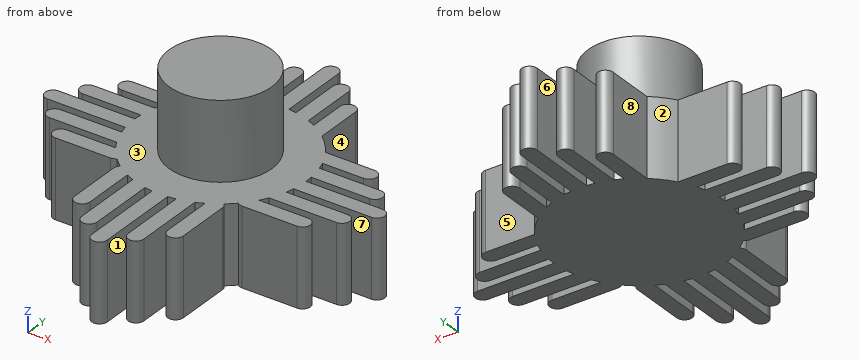
```python
from build123d import *

# Parameters (mm, degrees)
BOSS_EXTRUDE3_DEPTH    = 10
BOSS_EXTRUDE3_2_DEPTH  = 10
BOSS_EXTRUDE3_3_DEPTH  = 10
BOSS_EXTRUDE3_4_DEPTH  = 10
BOSS_EXTRUDE3_5_DEPTH  = 10
BOSS_EXTRUDE3_6_DEPTH  = 10
BOSS_EXTRUDE3_7_DEPTH  = 10
BOSS_EXTRUDE3_8_DEPTH  = 10
BOSS_EXTRUDE3_9_DEPTH  = 10
BOSS_EXTRUDE3_10_DEPTH = 10
BOSS_EXTRUDE3_11_DEPTH = 10
BOSS_EXTRUDE3_12_DEPTH = 10
BOSS_EXTRUDE3_13_DEPTH = 10
BOSS_EXTRUDE3_14_DEPTH = 10
BOSS_EXTRUDE3_15_DEPTH = 10
BOSS_EXTRUDE3_16_DEPTH = 10
BOSS_EXTRUDE3_17_DEPTH = 10
BOSS_EXTRUDE3_18_DEPTH = 10
BOSS_EXTRUDE3_19_DEPTH = 10
BOSS_EXTRUDE3_20_DEPTH = 10
SKETCH12_R             = 11
BOSS_EXTRUDE4_DEPTH    = 10
SKETCH13_R             = 6.585
BOSS_EXTRUDE5_DEPTH    = 10


with BuildPart() as part:
    # Sketch11 → Boss-Extrude3 (new body)
    with BuildSketch(Plane.XY):
        with BuildLine():
            Line((24.4, 31.507143862), (24.4, 46.249205315))
            ThreePointArc((24.4, 46.249205315), (25.4, 47.249205315), (26.4, 46.249205315))
            Line((26.4, 46.249205315), (26.4, 31.507143862))
            ThreePointArc((26.4, 31.507143862), (25.4, 30.507143862), (24.4, 31.507143862))
        make_face()
    extrude(amount=BOSS_EXTRUDE3_DEPTH)



with BuildPart() as body_2:
    # Sketch11 → Boss-Extrude3 2 (new body)
    with BuildSketch(Plane.XY):
        with BuildLine():
            Line((27.4, 30.400840206), (27.4, 43.867696771))
            ThreePointArc((27.4, 43.867696771), (28.4, 44.867696771), (29.4, 43.867696771))
            Line((29.4, 43.867696771), (29.4, 30.400840206))
            ThreePointArc((29.4, 30.400840206), (28.4, 29.400840206), (27.4, 30.400840206))
        make_face()
    extrude(amount=BOSS_EXTRUDE3_2_DEPTH)


with BuildPart() as body_3:
    # Sketch11 → Boss-Extrude3 3 (new body)
    with BuildSketch(Plane.XY):
        with BuildLine():
            Line((30.4, 33.885281374), (30.4, 40.954829552))
            ThreePointArc((30.4, 40.954829552), (31.4, 41.954829552), (32.4, 40.954829552))
            Line((32.4, 40.954829552), (32.4, 33.885281374))
            ThreePointArc((32.4, 33.885281374), (31.4, 32.885281374), (30.4, 33.885281374))
        make_face()
    extrude(amount=BOSS_EXTRUDE3_3_DEPTH)


with BuildPart() as body_4:
    # Sketch11 → Boss-Extrude3 4 (new body)
    with BuildSketch(Plane.XY):
        with BuildLine():
            Line((23.4, 30.400840206), (23.4, 43.867696771))
            ThreePointArc((23.4, 43.867696771), (22.4, 44.867696771), (21.4, 43.867696771))
            Line((21.4, 43.867696771), (21.4, 30.400840206))
            ThreePointArc((21.4, 30.400840206), (22.4, 29.400840206), (23.4, 30.400840206))
        make_face()
    extrude(amount=BOSS_EXTRUDE3_4_DEPTH)


with BuildPart() as body_5:
    # Sketch11 → Boss-Extrude3 5 (new body)
    with BuildSketch(Plane.XY):
        with BuildLine():
            Line((20.4, 33.885281374), (20.4, 40.954829552))
            ThreePointArc((20.4, 40.954829552), (19.4, 41.954829552), (18.4, 40.954829552))
            Line((18.4, 40.954829552), (18.4, 33.885281374))
            ThreePointArc((18.4, 33.885281374), (19.4, 32.885281374), (20.4, 33.885281374))
        make_face()
    extrude(amount=BOSS_EXTRUDE3_5_DEPTH)


with BuildPart() as body_6:
    # Sketch11 → Boss-Extrude3 6 (new body)
    with BuildSketch(Plane.XY):
        with BuildLine():
            Line((31.507143862, 26.4), (46.249205315, 26.4))
            ThreePointArc((46.249205315, 26.4), (47.249205315, 25.4), (46.249205315, 24.4))
            Line((46.249205315, 24.4), (31.507143862, 24.4))
            ThreePointArc((31.507143862, 24.4), (30.507143862, 25.4), (31.507143862, 26.4))
        make_face()
    extrude(amount=BOSS_EXTRUDE3_6_DEPTH)


with BuildPart() as body_7:
    # Sketch11 → Boss-Extrude3 7 (new body)
    with BuildSketch(Plane.XY):
        with BuildLine():
            Line((30.400840206, 23.4), (43.867696771, 23.4))
            ThreePointArc((43.867696771, 23.4), (44.867696771, 22.4), (43.867696771, 21.4))
            Line((43.867696771, 21.4), (30.400840206, 21.4))
            ThreePointArc((30.400840206, 21.4), (29.400840206, 22.4), (30.400840206, 23.4))
        make_face()
    extrude(amount=BOSS_EXTRUDE3_7_DEPTH)


with BuildPart() as body_8:
    # Sketch11 → Boss-Extrude3 8 (new body)
    with BuildSketch(Plane.XY):
        with BuildLine():
            Line((33.885281374, 20.4), (40.954829552, 20.4))
            ThreePointArc((40.954829552, 20.4), (41.954829552, 19.4), (40.954829552, 18.4))
            Line((40.954829552, 18.4), (33.885281374, 18.4))
            ThreePointArc((33.885281374, 18.4), (32.885281374, 19.4), (33.885281374, 20.4))
        make_face()
    extrude(amount=BOSS_EXTRUDE3_8_DEPTH)


with BuildPart() as body_9:
    # Sketch11 → Boss-Extrude3 9 (new body)
    with BuildSketch(Plane.XY):
        with BuildLine():
            Line((30.400840206, 27.4), (43.867696771, 27.4))
            ThreePointArc((43.867696771, 27.4), (44.867696771, 28.4), (43.867696771, 29.4))
            Line((43.867696771, 29.4), (30.400840206, 29.4))
            ThreePointArc((30.400840206, 29.4), (29.400840206, 28.4), (30.400840206, 27.4))
        make_face()
    extrude(amount=BOSS_EXTRUDE3_9_DEPTH)


with BuildPart() as body_10:
    # Sketch11 → Boss-Extrude3 10 (new body)
    with BuildSketch(Plane.XY):
        with BuildLine():
            Line((33.885281374, 30.4), (40.954829552, 30.4))
            ThreePointArc((40.954829552, 30.4), (41.954829552, 31.4), (40.954829552, 32.4))
            Line((40.954829552, 32.4), (33.885281374, 32.4))
            ThreePointArc((33.885281374, 32.4), (32.885281374, 31.4), (33.885281374, 30.4))
        make_face()
    extrude(amount=BOSS_EXTRUDE3_10_DEPTH)


with BuildPart() as body_11:
    # Sketch11 → Boss-Extrude3 11 (new body)
    with BuildSketch(Plane.XY):
        with BuildLine():
            Line((26.4, 19.292856138), (26.4, 4.550794685))
            ThreePointArc((26.4, 4.550794685), (25.4, 3.550794685), (24.4, 4.550794685))
            Line((24.4, 4.550794685), (24.4, 19.292856138))
            ThreePointArc((24.4, 19.292856138), (25.4, 20.292856138), (26.4, 19.292856138))
        make_face()
    extrude(amount=BOSS_EXTRUDE3_11_DEPTH)


with BuildPart() as body_12:
    # Sketch11 → Boss-Extrude3 12 (new body)
    with BuildSketch(Plane.XY):
        with BuildLine():
            Line((23.4, 20.399159794), (23.4, 6.932303229))
            ThreePointArc((23.4, 6.932303229), (22.4, 5.932303229), (21.4, 6.932303229))
            Line((21.4, 6.932303229), (21.4, 20.399159794))
            ThreePointArc((21.4, 20.399159794), (22.4, 21.399159794), (23.4, 20.399159794))
        make_face()
    extrude(amount=BOSS_EXTRUDE3_12_DEPTH)


with BuildPart() as body_13:
    # Sketch11 → Boss-Extrude3 13 (new body)
    with BuildSketch(Plane.XY):
        with BuildLine():
            Line((20.4, 16.914718626), (20.4, 9.845170448))
            ThreePointArc((20.4, 9.845170448), (19.4, 8.845170448), (18.4, 9.845170448))
            Line((18.4, 9.845170448), (18.4, 16.914718626))
            ThreePointArc((18.4, 16.914718626), (19.4, 17.914718626), (20.4, 16.914718626))
        make_face()
    extrude(amount=BOSS_EXTRUDE3_13_DEPTH)


with BuildPart() as body_14:
    # Sketch11 → Boss-Extrude3 14 (new body)
    with BuildSketch(Plane.XY):
        with BuildLine():
            Line((27.4, 20.399159794), (27.4, 6.932303229))
            ThreePointArc((27.4, 6.932303229), (28.4, 5.932303229), (29.4, 6.932303229))
            Line((29.4, 6.932303229), (29.4, 20.399159794))
            ThreePointArc((29.4, 20.399159794), (28.4, 21.399159794), (27.4, 20.399159794))
        make_face()
    extrude(amount=BOSS_EXTRUDE3_14_DEPTH)


with BuildPart() as body_15:
    # Sketch11 → Boss-Extrude3 15 (new body)
    with BuildSketch(Plane.XY):
        with BuildLine():
            Line((30.4, 16.914718626), (30.4, 9.845170448))
            ThreePointArc((30.4, 9.845170448), (31.4, 8.845170448), (32.4, 9.845170448))
            Line((32.4, 9.845170448), (32.4, 16.914718626))
            ThreePointArc((32.4, 16.914718626), (31.4, 17.914718626), (30.4, 16.914718626))
        make_face()
    extrude(amount=BOSS_EXTRUDE3_15_DEPTH)


with BuildPart() as body_16:
    # Sketch11 → Boss-Extrude3 16 (new body)
    with BuildSketch(Plane.XY):
        with BuildLine():
            Line((19.292856138, 24.4), (4.550794685, 24.4))
            ThreePointArc((4.550794685, 24.4), (3.550794685, 25.4), (4.550794685, 26.4))
            Line((4.550794685, 26.4), (19.292856138, 26.4))
            ThreePointArc((19.292856138, 26.4), (20.292856138, 25.4), (19.292856138, 24.4))
        make_face()
    extrude(amount=BOSS_EXTRUDE3_16_DEPTH)


with BuildPart() as body_17:
    # Sketch11 → Boss-Extrude3 17 (new body)
    with BuildSketch(Plane.XY):
        with BuildLine():
            Line((20.399159794, 27.4), (6.932303229, 27.4))
            ThreePointArc((6.932303229, 27.4), (5.932303229, 28.4), (6.932303229, 29.4))
            Line((6.932303229, 29.4), (20.399159794, 29.4))
            ThreePointArc((20.399159794, 29.4), (21.399159794, 28.4), (20.399159794, 27.4))
        make_face()
    extrude(amount=BOSS_EXTRUDE3_17_DEPTH)


with BuildPart() as body_18:
    # Sketch11 → Boss-Extrude3 18 (new body)
    with BuildSketch(Plane.XY):
        with BuildLine():
            Line((16.914718626, 30.4), (9.845170448, 30.4))
            ThreePointArc((9.845170448, 30.4), (8.845170448, 31.4), (9.845170448, 32.4))
            Line((9.845170448, 32.4), (16.914718626, 32.4))
            ThreePointArc((16.914718626, 32.4), (17.914718626, 31.4), (16.914718626, 30.4))
        make_face()
    extrude(amount=BOSS_EXTRUDE3_18_DEPTH)


with BuildPart() as body_19:
    # Sketch11 → Boss-Extrude3 19 (new body)
    with BuildSketch(Plane.XY):
        with BuildLine():
            Line((20.399159794, 23.4), (6.932303229, 23.4))
            ThreePointArc((6.932303229, 23.4), (5.932303229, 22.4), (6.932303229, 21.4))
            Line((6.932303229, 21.4), (20.399159794, 21.4))
            ThreePointArc((20.399159794, 21.4), (21.399159794, 22.4), (20.399159794, 23.4))
        make_face()
    extrude(amount=BOSS_EXTRUDE3_19_DEPTH)


with BuildPart() as body_20:
    # Sketch11 → Boss-Extrude3 20 (new body)
    with BuildSketch(Plane.XY):
        with BuildLine():
            Line((16.914718626, 20.4), (9.845170448, 20.4))
            ThreePointArc((9.845170448, 20.4), (8.845170448, 19.4), (9.845170448, 18.4))
            Line((9.845170448, 18.4), (16.914718626, 18.4))
            ThreePointArc((16.914718626, 18.4), (17.914718626, 19.4), (16.914718626, 20.4))
        make_face()
    extrude(amount=BOSS_EXTRUDE3_20_DEPTH)


with BuildPart() as part_1:
    add(part.part)

    add(body_2.part)  # Boss-Extrude4 merges body 2

    add(body_3.part)  # Boss-Extrude4 merges body 3

    add(body_4.part)  # Boss-Extrude4 merges body 4

    add(body_5.part)  # Boss-Extrude4 merges body 5

    add(body_6.part)  # Boss-Extrude4 merges body 6

    add(body_7.part)  # Boss-Extrude4 merges body 7

    add(body_8.part)  # Boss-Extrude4 merges body 8

    add(body_9.part)  # Boss-Extrude4 merges body 9

    add(body_10.part)  # Boss-Extrude4 merges body 10

    add(body_11.part)  # Boss-Extrude4 merges body 11

    add(body_12.part)  # Boss-Extrude4 merges body 12

    add(body_13.part)  # Boss-Extrude4 merges body 13

    add(body_14.part)  # Boss-Extrude4 merges body 14

    add(body_15.part)  # Boss-Extrude4 merges body 15

    add(body_16.part)  # Boss-Extrude4 merges body 16

    add(body_17.part)  # Boss-Extrude4 merges body 17

    add(body_18.part)  # Boss-Extrude4 merges body 18

    add(body_19.part)  # Boss-Extrude4 merges body 19

    add(body_20.part)  # Boss-Extrude4 merges body 20
    # Sketch12 → Boss-Extrude4 (add)
    with BuildSketch(Plane.XY):
        with Locations((25.4, 26.4)):
            Circle(SKETCH12_R)
    extrude(amount=BOSS_EXTRUDE4_DEPTH)

    # Sketch13 → Boss-Extrude5 (add)
    with BuildSketch(Plane.XY.offset(10)):
        with Locations((25.4, 26.4)):
            Circle(SKETCH13_R)
    extrude(amount=BOSS_EXTRUDE5_DEPTH)


solid = part_1.part
```
Source: CAD feature listing. Evaluate the final solid. Frame: model axes, mm. Face numbers are marked on the shaded views. A direction names the side the tool comes from. Give positions to 0.01 mm unless a question says otherwise; leave off trailing zeros. Loops run counter-clockwise (first coordinate to the right, second up) from the corner with the lowest first, then second, coordinate; pieces in that order, holes last. Notation, with made-up numbers: M 80,80.25 L 138,80.25 A18 ccw 138,104.25 Z; hole C 79,-34 d6. An arc over 180 degrees is marked long. Put each result on its own line as item: value.
Q1. Reachability of the marked faces 5, 6, 7 and 8 from +Z, -Z, +X, -X, +Y, -Y: full face, straight path, thin tool, end or side. Return the list, or none.
Response values:
face 5: +Z, -Z, +X, +Y
face 6: +Z, -Z, +Y
face 7: +Z, -Z, +X
face 8: +Z, -Z, -X, +Y
Q2. Section B-B (y = 25.4). Return the cut outline in (x, z), and give its area (3 significant figures).
Response values:
outline: M 3.55,0 L 47.25,0 L 47.25,10 L 31.91,10 L 31.91,20 L 18.89,20 L 18.89,10 L 3.55,10 Z
area: 567 mm²
Q3. Mould query, pull axis X, two halves, no side actions, for the marked faces 1, 2, 3 and 4. Classes: released by +X, released by -X, zero draft, split by the parting line, or undercut.
Response values:
face 1: undercut
face 2: released by -X
face 3: zero draft
face 4: released by +X
Q4. Section A-A (x = 12). Return the cut outline in (y, z), and give its area (3 significant figures).
Response values:
outline: M 18.4,0 L 20.4,0 L 20.4,10 L 18.4,10 Z; M 21.4,0 L 23.4,0 L 23.4,10 L 21.4,10 Z; M 24.4,0 L 26.4,0 L 26.4,10 L 24.4,10 Z; M 27.4,0 L 29.4,0 L 29.4,10 L 27.4,10 Z; M 30.4,0 L 32.4,0 L 32.4,10 L 30.4,10 Z
area: 100 mm²
Q5. Pin query (flat end, axial travel): P1, Ø1.5, axis at y = 17.5, z = 10, coming from the +X side; P2, Ø6, axis at y = 21, z = 9.5, coming from the -X side; P3, Ø8, axis at x = 35, y = 34, coming from the -Z side; P4, Ø8, axis at y = 7.5, z = 4, coming from the +X side. Return the tip coordinate at first contact, or that it passes through.
Response values:
P1: stops at x = 32.79
P2: stops at x = 5.93
P3: stops at z = 0
P4: stops at x = 32.4
Q6. Section C-C (x = 19.4). Return the cut outline in (y, z).
Response values:
outline: M 8.85,0 L 41.95,0 L 41.95,10 L 29.11,10 L 29.11,20 L 23.69,20 L 23.69,10 L 8.85,10 Z
Q7. Line query: probe 1 along Y at (x, z) = (12.5, 5.75); probe 2 along X at (y, z) = (42.5, 2.5); probe 3 along X at (y, z) = (16, 8.25). Output: solid intervals per line, ascending. Write a range as [from, to].
Response values:
probe 1: y = [18.4, 20.4], [21.4, 23.4], [24.4, 26.4], [27.4, 29.4], [30.4, 32.4]
probe 2: x = [21.4, 23.4], [24.4, 26.4], [27.4, 29.4]
probe 3: x = [18.4, 20.4], [21.4, 29.4], [30.4, 32.4]
